Autodesk Inventor part; units mm, degrees
ref_plane "YZ Plane" through (0, 0, 0) normal (1, 0, 0) x (0, 1, 0)
ref_plane "XZ Plane" through (0, 0, 0) normal (0, 1, 0) x (-1, 0, 0)
ref_plane "XY Plane" through (0, 0, 0) normal (0, 0, 1) x (1, 0, 0)
sketch "Sketch1" plane through (0, 0, 0) normal (0, 1, 0) x (-1, 0, 0)
  line L0 (0, 0) -> (0, 300)
  line L1 (0, 300) -> (350, 300)
  line L2 (350, 300) -> (1000, 100)
  line L3 (0, 0) -> (1000, 0)
  line L4 (1000, 100) -> (1000, 0)
  line L5 (0, 0) -> (0, -300)
  line L6 (0, -300) -> (350, -300)
  line L7 (350, -300) -> (1000, -100)
  line L8 (1000, -100) -> (1000, 0)
  line L9 (350, 300) -> (350, -300)
  dimension "d12" = 300
  dimension "d13" = 350
  dimension "d16" = 100
extrude "Extrusion1" add sketch "Sketch1" along normal blind 20
fillet "Fillet1" radius 50 1 edges at (-1000, 10, 100)
fillet "Fillet2" radius 50 1 edges at (-1000, 10, -100)
chamfer "Chamfer1" distance 40 angle 45 1 edges at (0, 10, -300)
chamfer "Chamfer2" distance 40 angle 45 1 edges at (0, 10, 300)
sketch "Sketch3" plane through (0, 20, 0) normal (0, 1, 0) x (1, 0, 0)
  point P0 (0, 0)
sketch "Sketch4" plane through (0, 20, 0) normal (0, 1, 0) x (1, 0, 0)
  point P0 (0, 0)
sketch "Sketch5" plane through (0, 20, 0) normal (0, 1, 0) x (1, 0, 0)
  line L0 (-780, 0) -> (-720, 0) construction
  line L1 (-762.5, -17.5) -> (-737.5, -17.5)
  line L2 (-737.5, 17.5) -> (-762.5, 17.5)
  arc A0 (-762.5, 17.5) -> (-762.5, -17.5) centre (-762.5, 0) ccw
  arc A1 (-737.5, -17.5) -> (-737.5, 17.5) centre (-737.5, 0) ccw
  line L3 (-1000, 63.0713) -> (-1000, -63.0713)
  point P0 (0, 0)
  point P1 (-750, 0)
  dimension "d27" = 60
  dimension "d28" = 35
extrude "Extrusion2" cut sketch "Sketch5" against normal blind 20
sketch "Sketch6" plane through (0, 20, 0) normal (0, 1, 0) x (1, 0, 0)
  line L0 (-1000, 63.0713) -> (-1000, -63.0713)
  line L1 (-1000, 0) -> (-950, 0)
  point P0 (0, 0)
  dimension "d33" = 50
hole "Hole1" at (-950, 20, 0) direction (0, -1, 0) diameter 10 end through all
sketch "Sketch7" plane through (0, 0, 0) normal (0, -1, 0) x (1, 0, 0)
  line L0 (-350, 300) -> (-40, 300)
  line L1 (0, -260) -> (-40, -300)
  line L2 (-40, 300) -> (-40, -300)
  line L3 (-40, -300) -> (-140, -300)
  line L4 (-140, -300) -> (-140, 300)
  line L5 (-140, 300) -> (-40, 300)
  point P0 (0, 0)
  dimension "d41" = 100
extrude "Extrusion3" add sketch "Sketch7" along normal blind 40
sketch "Sketch8" plane through (0, -40, 0) normal (0, -1, 0) x (1, 0, 0)
  line L0 (-350, 300) -> (-40, 300)
  circle A0 centre (-91.5513, 150) radius 5
  line L1 (-40, -300) -> (-40, 300)
  line L2 (-40, 0) -> (-140, 0)
  line L3 (-140, -300) -> (-140, 300)
  circle A1 centre (-91.5513, -150) radius 5
  point P0 (0, 0)
  dimension "d45" = 10
extrude "Extrusion4" cut sketch "Sketch8" against normal blind 60 contours A0 | A1
sketch "Sketch9" plane through (0, -40, 0) normal (0, -1, 0) x (1, 0, 0)
  line L0 (-40, -300) -> (-350, -300)
  line L1 (-139.5196, -300) -> (-39.5196, -300)
  line L2 (-39.5196, -300) -> (-39.5196, -250)
  line L3 (-39.5196, -250) -> (-139.5196, -250)
  line L4 (-139.5196, -250) -> (-139.5196, -300)
  line L5 (-40, -300) -> (-40, 300)
  line L6 (-40, 0) -> (-139.5196, 0)
  line L7 (-40, 300) -> (-350, 300)
  line L8 (-39.5196, 300) -> (-39.5196, 250)
  line L9 (-39.5196, 250) -> (-139.5196, 250)
  line L10 (-139.5196, 250) -> (-139.5196, 300)
  point P0 (0, 0)
  point P1 (-40, 250)
  point P2 (-40, -250)
  dimension "d48" = 100
  dimension "d49" = 50
extrude "Extrusion5" cut sketch "Sketch9" against normal blind 60 contours L0 L4 L3 L5 | L9 L10 L7 L5
sketch "Sketch10" plane through (0, 20, 0) normal (0, 1, 0) x (1, 0, 0)
  line L0 (-350, 300) -> (-964.7043, 110.8602)
  line L1 (-964.7043, 110.8602) -> (-764.7043, 110.8602)
  line L2 (-764.7043, 110.8602) -> (-350, 300)
  line L3 (-964.7043, -110.8602) -> (-350, -300)
  line L4 (-964.7043, -110.8602) -> (-764.7043, -110.8602)
  line L5 (-764.7043, -110.8602) -> (-350, -300)
  point P0 (0, 0)
  dimension "d53" = 200
extrude "Extrusion6" cut sketch "Sketch10" against normal blind 20
sketch "Sketch11" plane through (-139.5196, -40, 300) normal (1, 0, 0) x (0, 0, -1)
  line L0 (600, 40) -> (0, 40)
  line L1 (0, 40) -> (50, 40)
  line L2 (50, 0) -> (50, 60)
  line L3 (50, 0) -> (50, 40)
  line L4 (0, 0) -> (600, 0)
  line L5 (0, 40) -> (0, 0)
  line L6 (0, 0) -> (50, 0)
  point P0 (300, 40)
extrude "Extrusion7" cut sketch "Sketch11" against normal blind 1
sketch "Sketch12" plane through (-139.5196, -40, -250) normal (1, 0, 0) x (0, 0, -1)
  line L0 (50, 0) -> (0, 0)
  line L1 (0, 0) -> (0, 40)
  line L2 (50, 0) -> (0, 0)
  line L3 (0, 0) -> (0, 40)
  line L4 (0, 40) -> (50, 40)
  line L5 (50, 40) -> (50, 0)
  point P0 (-250, 40)
extrude "Extrusion8" cut sketch "Sketch12" against normal blind 1
properties part number "Base"
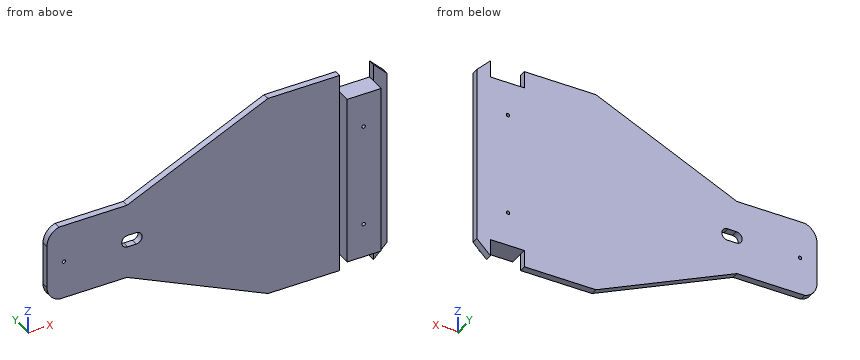
CAD build for the part. Positions are in the model's coordinates, mm. Give positions to 0.01 mm unless a question says otherwise; leave off trailing zeros. Write each loop counter-clockwise with the first axis right and the second up, starting at its lowest first coordinate (ties: lowest second). Pieces come first, ordered by that corner, then holes. Notation, with made-up numbers: (85, 52.5) -> (135, 52.5) arc R35 cw to (135, 90.5) -> close; hole circle Ø5 at (80, 16.5). An arc over 180 degrees is marked (long way). Write each question's results on one line, items separated by ' | '.
1. Cut at A-A, the plane z = 44. Write the cut outline in (x, y).
Geometry check:
outline: (-1000, 0) -> (-140, 0) -> (-140, -40) -> (-40, -40) -> (-40, 0) -> (0, 0) -> (0, 20) -> (-1000, 20) -> close
2. Cut at D-D, the plane z = 204.5. Write the cut outline in (x, y).
Geometry check:
outline: (-559.39, 0) -> (-140, 0) -> (-140, -40) -> (-40, -40) -> (-40, 0) -> (0, 0) -> (0, 20) -> (-559.39, 20) -> close
3. Cut at C-C, the plane x = -893.5. Write the cut outline in (y, z).
Geometry check:
outline: (0, -110.86) -> (20, -110.86) -> (20, 110.86) -> (0, 110.86) -> close
4. Cut at B-B, the plane x = -223. Write the cut outline in (y, z).
Geometry check:
outline: (0, -300) -> (20, -300) -> (20, 300) -> (0, 300) -> close
5. Drop flat-ended pins along their axis: P1, Ø10, axis at x = -902, y = 12.5, coming from the -Z side; P2, Ø16, axis at x = -950, z = 0, coming from the -Y side; P3, Ø1.5, axis at x = -838, y = -2, coming from the +Z side; P4, Ø20, axis at y = -11.5, z = 19, coming from the -X side. Give the stop position or say it passes through.
Geometry check:
P1: z = -110.86 | P2: y = 0 | P3: through | P4: x = -140
6. Wall check: probe 1 along X at (y, z) = (7, 0); probe 2 along Z at (x, y) = (-950, 6.5); probe 3 along X at (y, z) = (-33, 47). Give the ranges that are in metal, low to high. Write a range as [from, to].
Geometry check:
probe 1: [-1000, -955], [-945, -780], [-720, 0] | probe 2: [-110.86, -5], [5, 110.86] | probe 3: [-140, -40]
